```python
from build123d import *

# Parameters (mm, degrees)
SKETCH1_W           = 76.2
SKETCH1_H           = 53.594
SKETCH1_R           = 3.175
SKETCH1_W_2         = 38.1
SKETCH1_H_2         = 127
BOSS_EXTRUDE1_DEPTH = 0.79375
SKETCH2_R           = 2.5527
SKETCH2_R_2         = 1.9812
CUT_EXTRUDE1_DEPTH  = 115.487259799
CUT_EXTRUDE2_DEPTH  = 115.487259799
FILLET2_R           = 1.5875
CHAMFER1_SIZE       = 4.7625
FILLET3_R           = 3.175
CUT_EXTRUDE3_DEPTH  = 115.487259799
FILLET5_R           = 1.5875


with BuildPart() as part:
    # Sketch1 → Boss-Extrude1 (new, symmetric)
    # profile 1 of 2: a face of its own
    with BuildSketch(Plane.XY):
        with Locations((57.15, -1.778)):
            Rectangle(SKETCH1_W, SKETCH1_H)
        with Locations((32.1437, -15.875)):
            Circle(SKETCH1_R, mode=Mode.SUBTRACT)
        with Locations((88.9, 12.319)):
            Circle(SKETCH1_R, mode=Mode.SUBTRACT)
    # profile 2 of 2: a face of its own
    with BuildSketch(Plane.XY):
        Rectangle(SKETCH1_W_2, SKETCH1_H_2)
    extrude(amount=BOSS_EXTRUDE1_DEPTH, both=True)

    # Sketch2 → Cut-Extrude1 (cut, through all)
    with BuildSketch(Plane.XY.offset(0.79375)):
        with Locations((-12.7, -57.15)):
            Circle(SKETCH2_R)
        with Locations((12.7, -57.15)):
            Circle(SKETCH2_R)
        with Locations((0, -31.75)):
            Circle(SKETCH2_R)
        with Locations((0, -9.8425)):
            Circle(SKETCH2_R_2)
        with Locations((0, 9.2075)):
            Circle(SKETCH2_R_2)
        with Locations((0, 39.6875)):
            Circle(SKETCH2_R_2)
        with Locations((0, 58.7375)):
            Circle(SKETCH2_R_2)
    extrude(amount=-CUT_EXTRUDE1_DEPTH, mode=Mode.SUBTRACT)

    # Sketch3 → Cut-Extrude2 (cut, through all)
    with BuildSketch(Plane.XY.offset(0.79375)):
        Polygon((45.671811727, 9.144), (60.52185, 1.767162907), (75.371888273, 9.144), align=None)
        Polygon((35.3187, 7.196638614), (35.3187, -10.752638614), (53.385213498, -1.778), align=None)
        Polygon((60.52185, -5.323162907), (45.671811727, -12.7), (75.371888273, -12.7), align=None)
        Polygon((85.725, 7.196638614), (67.658486502, -1.778), (85.725, -10.752638614), align=None)
    extrude(amount=-CUT_EXTRUDE2_DEPTH, mode=Mode.SUBTRACT)

    # Fillet2
    fillet2_edges = [part.edges().sort_by_distance(p)[0] for p in [
        (60.52185, 1.767162907, 0),
        (45.671811727, 9.144, 0),
        (75.371888273, 9.144, 0),
        (35.3187, -10.752638614, 0),
        (35.3187, 7.196638614, 0),
        (53.385213498, -1.778, 0),
        (45.671811727, -12.7, 0),
        (60.52185, -5.323162907, 0),
        (75.371888273, -12.7, 0),
        (67.658486502, -1.778, 0),
        (85.725, 7.196638614, 0),
        (85.725, -10.752638614, 0),
    ]]
    fillet(fillet2_edges, radius=FILLET2_R)

    # Chamfer1
    chamfer1_edges = [part.edges().sort_by_distance(p)[0] for p in [
        (95.25, -28.575, 0),
        (19.05, -63.5, 0),
        (-19.05, -63.5, 0),
        (-19.05, 63.5, 0),
        (19.05, 63.5, 0),
        (95.25, 25.019, 0),
    ]]
    chamfer(chamfer1_edges, length=CHAMFER1_SIZE)

    # Fillet3
    fillet3_edges = [part.edges().sort_by_distance(p)[0] for p in [
        (19.05, -28.575, 0),
        (90.4875, 25.019, 0),
        (19.05, 25.019, 0),
        (95.25, -23.8125, 0),
        (95.25, 20.2565, 0),
        (90.4875, -28.575, 0),
        (19.05, -58.7375, 0),
        (-14.2875, -63.5, 0),
        (14.2875, -63.5, 0),
        (-19.05, 58.7375, 0),
        (-19.05, -58.7375, 0),
        (-14.2875, 63.5, 0),
        (14.2875, 63.5, 0),
        (19.05, 58.7375, 0),
    ]]
    fillet(fillet3_edges, radius=FILLET3_R)

    # Sketch5 → Cut-Extrude3 (cut, through all)
    with BuildSketch(Plane.XY.offset(0.79375)):
        with BuildLine():
            ThreePointArc((-6.35, -24.650484171), (0, -22.225), (6.35, -24.650484171))
            Line((6.35, -24.650484171), (6.35, -14.605))
            ThreePointArc((6.35, -14.605), (0, -17.78), (-6.35, -14.605))
            Line((-6.35, -14.605), (-6.35, -24.650484171))
        make_face()
        with BuildLine():
            Line((6.35, -5.08), (6.35, 4.445))
            ThreePointArc((6.35, 4.445), (0, 1.27), (-6.35, 4.445))
            Line((-6.35, 4.445), (-6.35, -5.08))
            ThreePointArc((-6.35, -5.08), (0, -1.905), (6.35, -5.08))
        make_face()
        with BuildLine():
            Line((6.35, 13.97), (6.35, 28.194))
            Line((6.35, 28.194), (6.35, 32.587984171))
            ThreePointArc((6.35, 32.587984171), (0, 30.1625), (-6.35, 32.587984171))
            Line((-6.35, 32.587984171), (-6.35, 13.97))
            ThreePointArc((-6.35, 13.97), (0, 17.145), (6.35, 13.97))
        make_face()
    extrude(amount=-CUT_EXTRUDE3_DEPTH, mode=Mode.SUBTRACT)

    # Fillet5
    fillet5_edges = [part.edges().sort_by_distance(p)[0] for p in [
        (6.35, -24.650484171, 0),
        (-6.35, -24.650484171, 0),
        (-6.35, -14.605, 0),
        (6.35, -14.605, 0),
        (6.35, -5.08, 0),
        (-6.35, -5.08, 0),
        (-6.35, 4.445, 0),
        (6.35, 4.445, 0),
        (6.35, 13.97, 0),
        (-6.35, 13.97, 0),
        (-6.35, 32.587984171, 0),
        (6.35, 32.587984171, 0),
    ]]
    fillet(fillet5_edges, radius=FILLET5_R)


solid = part.part
```
Design review of the part built by this model. Coordinates are the model's own, in mm. A direction names the side the tool comes from. Coordinates: 2 decimals unless noted, no trailing zeros. Order: outer loops, then holes, each group sorted by start corner. A loop starts at its lowest first (then second) coordinate and runs counter-clockwise, first axis right, second up. Notation, with made-up numbers: (78.5, 89.25) - (90.5, 89.25) arc R20 ccw to (90.5, 95.25) - close; hole circle Ø2 at (-23, 71.25). An arc over 180 degrees is marked (long way). One line per question, with ' | ' between items.
Q1. Consider section A-A, the plane x = 57.5. Give the boundary of the cut face in (y, z) (3 decimals).
Answer key:
outline: (-28.575, -0.794) - (-12.7, -0.794) - (-12.7, 0.794) - (-28.575, 0.794) - close; (-6.824, -0.794) - (3.268, -0.794) - (3.268, 0.794) - (-6.824, 0.794) - close; (9.144, -0.794) - (25.019, -0.794) - (25.019, 0.794) - (9.144, 0.794) - close
Q2. To check wall thickness, follow line 1 along X through (y, z) = (-21.5, -0.55); line 2 along Y through (x, z) = (4, -0.2); line 3 along X through (y, z) = (-55.5, 0.7). State the ranges of each line that lie inside material, in increasing order.
Answer key:
line 1: x = -19.05 to -6.35, 6.35 to 95.25 | line 2: y = -63.5 to -23.11, -16.7 to -2.99, 2.35 to 16.06, 31.04 to 63.5 | line 3: x = -19.05 to -14.65, -10.75 to 10.75, 14.65 to 19.05
Q3. Consider section B-B, the plane x = 44. Give the boundary of the cut face in (y, z) (3 decimals), then the cut area to 3 significant figures.
Answer key:
outline: (-28.575, -0.794) - (-6.44, -0.794) - (-6.44, 0.794) - (-28.575, 0.794) - close; (2.884, -0.794) - (25.019, -0.794) - (25.019, 0.794) - (2.884, 0.794) - close | area: 70.3 mm2
Q4. Clearance check with flat-ended pins moving along their axes: pin 1 Ø0.8 at (y, z) = (49.5, 0) entering from +X; pin 2 Ø0.8 at (x, z) = (58, -0.5) entering from +Y; pin 3 Ø0.8 at (x, z) = (57, 0) entering from -Y (3 decimals). State where each tip first meets the part, or that it passes through.
Answer key:
pin 1: stops at x = 19.05 | pin 2: stops at y = 25.02 | pin 3: stops at y = -28.575
Q5. For faces 1 (the cylindrical face through (19.96, 25.97, -0.01)), 2 (the flat face through (65.33, -7.71, 0.01)), list the 3-axis set-ups (+Z, -Z, +X, -X, +Y, -Y) from which the entire face can be reached by the end or side of a thin tool; tool diameter is ignored.
Answer key:
face 1: +Z, -Z, +X, +Y | face 2: +Z, -Z
Q6. The part is to be moulded in two halves that separate along X. For faces 3 (the flat face through (43.98, -6.45, 0.01)), 4 (the cylindrical face through (19.955, -29.53, 0.011)), 5 (the flat face through (25, 1, 0.794)), say which applies: +X half, -X half, draft (parallel to the pull), parting line (faces both ways), or undercut.
Answer key:
face 3: undercut | face 4: +X half | face 5: draft
Q7. Consider section C-C, the plane x = 0. Give the number of separate pieces and of enclosed holes in the cut face, then the cut area to 3 significant figures.
Answer key:
separate pieces: 9 | enclosed holes: 0 | area: 136 mm2
